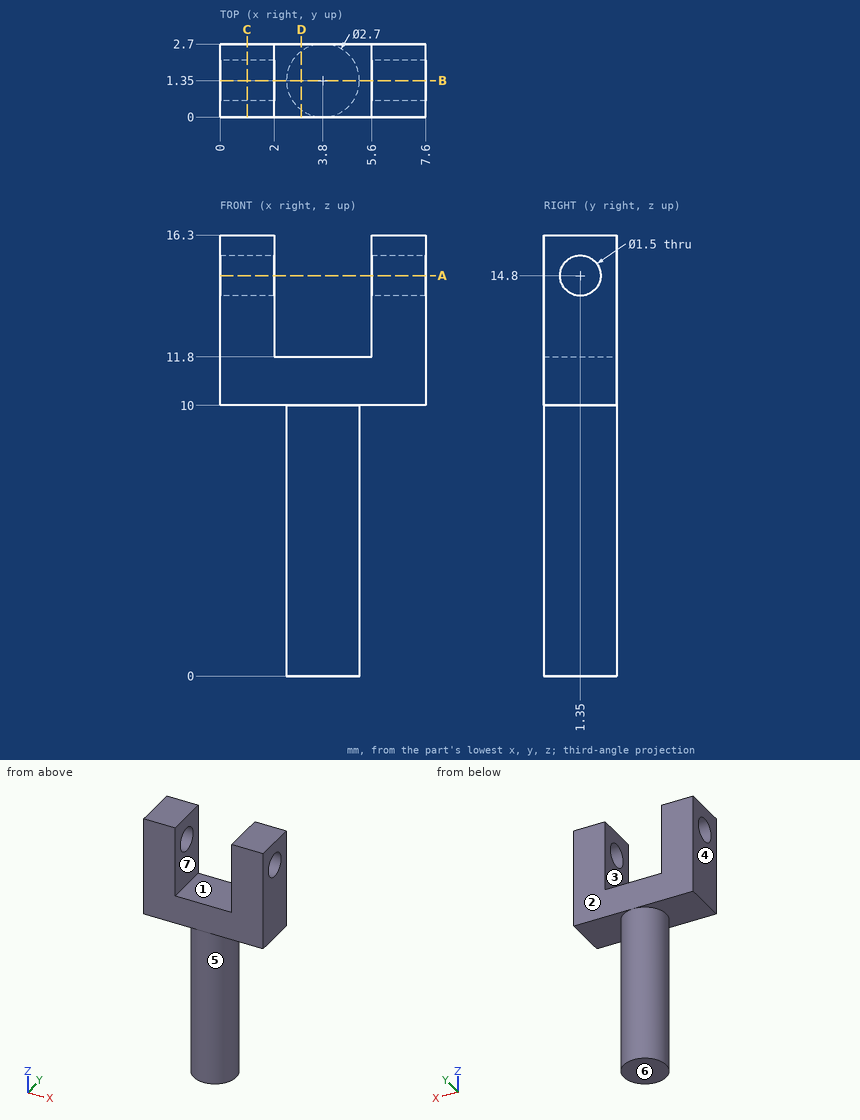
Here's the drawing with two shaded views (mm, measured from the low corner). I have some questions. A direction names the side the tool comes from. Give positions to 0.01 mm unless a question says otherwise; leave off trailing zeros. Order: outer loops, then holes, each group sorted by start corner. A loop starts at its lowest first (then second) coordinate and runs counter-clockwise, first axis right, second up. Notation, with made-up numbers: (-6, 79) - (18, 79) arc R10 ccw to (18, 96) - close; hole circle Ø10 at (66, 87.25). An arc over 180 degrees is marked (long way). Use a Markdown table: item, result. Add a question column.
Q1. If we section it at A-A on z = 14.8: Write out the boundary of the cut face in (x, y).
Q2. I'm going to push flat-ended pins straight in: pin 1 (1.5 mm diameter, centred on y = 1, z = 8, fed in from -X); pin 2 (1.5 mm diameter, centred on y = 1, z = 3, fed in from +X); pin 3 (0.8 mm diameter, centred on x = 5.5, y = 2, fed in from -Z); pin 4 (1.4 mm diameter, centred on y = 1.35, z = 14.8, fed in from +X). Where does each tip first touch, or does it pass through?
Q3. Please list where these lines run through material, in increasing order: line 1 along Y through (x, z) = (7.15, 14.8); line 2 along Z through (x, y) = (6.25, 1.4); line 3 along X through (y, z) = (0.35, 13.5).
Q4. On a 3-axis mill with a long thin cutter (end or side, diameter ignored), from which of +Z, -Z, +X, -X, +Y, -Y can I reach the whole of each face in a straight line? I mean the marked faces 5, 6 and 7. Say none if no direction works.
Q5. If we section it at C-C on x = 1: Write out the boundary of the cut face in (y, z).
Q6. If we section it at D-D on x = 3: Write out the boundary of the cut face in (y, z), plus the area to 3 significant figures.
Q7. If we section it at B-B on y = 1.35: Write out the boundary of the cut face in (x, z), plus the area to 3 significant figures.
Q8. If we mould it in two halves opening along X, with no side actions, what happens to the marked faces 1, 2, 3 and 4? For each: released by +X, released by -X, zero draft, split by the parting line, or undercut.
Answers follow:
| question | item | result |
|---|---|---|
| 1 | outline | (0, 0) - (2, 0) - (2, 0.6) - (0, 0.6) - close; (0, 2.1) - (2, 2.1) - (2, 2.7) - (0, 2.7) - close; (5.6, 0) - (7.6, 0) - (7.6, 0.6) - (5.6, 0.6) - close; (5.6, 2.1) - (7.6, 2.1) - (7.6, 2.7) - (5.6, 2.7) - close |
| 2 | pin 1 | stops at x = 2.45 |
| 2 | pin 2 | stops at x = 5.15 |
| 2 | pin 3 | stops at z = 10 |
| 2 | pin 4 | passes through |
| 3 | line 1 | y = 0 to 0.6, 2.1 to 2.7 |
| 3 | line 2 | z = 10 to 14.05, 15.55 to 16.3 |
| 3 | line 3 | x = 0 to 2, 5.6 to 7.6 |
| 4 | face 5 | -Z |
| 4 | face 6 | -Z, +X, -X, +Y, -Y |
| 4 | face 7 | +Z, +Y, -Y |
| 5 | outline | (0, 10) - (2.7, 10) - (2.7, 16.3) - (0, 16.3) - close; hole circle Ø1.5 at (1.35, 14.8) |
| 6 | outline | (0, 10) - (0.26, 10) - (0.26, 0) - (2.44, 0) - (2.44, 10) - (2.7, 10) - (2.7, 11.8) - (0, 11.8) - close |
| 6 | area | 26.6 mm^2 |
| 7 | outline | (0, 10) - (2.45, 10) - (2.45, 0) - (5.15, 0) - (5.15, 10) - (7.6, 10) - (7.6, 14.05) - (5.6, 14.05) - (5.6, 11.8) - (2, 11.8) - (2, 14.05) - (0, 14.05) - close; (0, 15.55) - (2, 15.55) - (2, 16.3) - (0, 16.3) - close; (5.6, 15.55) - (7.6, 15.55) - (7.6, 16.3) - (5.6, 16.3) - close |
| 7 | area | 52.7 mm^2 |
| 8 | face 1 | undercut |
| 8 | face 2 | zero draft |
| 8 | face 3 | undercut |
| 8 | face 4 | released by -X |
